Geometry check sheet. Reference: drawing and pictorial views, mm from the part's lowest x, y, z. A direction names the side the tool comes from. Coordinates: 2 decimals unless noted, no trailing zeros. Order: outer loops, then holes, each group sorted by start corner. A loop starts at its lowest first (then second) coordinate and runs counter-clockwise, first axis right, second up. Notation, with made-up numbers: (18.5, 58.25) -> (56.5, 58.25) arc R27 ccw to (56.5, 83.25) -> close; hole circle Ø4 at (75.25, 79). An arc over 180 degrees is marked (long way). Use CSV: the item, a comma, the result in double quotes. Start each with the question number.
1) Tool access check on the marked faces 1 and 2. Record the directions out of +Z, -Z, +X, -X, +Y, -Y that give a thin tool (end or side, any length) a straight path to the whole face; none if there is none.
2) Scan lines: line 1 along X through (y, z) = (6.25, 72) (3 decimals); line 2 along Z through (x, y) = (22.5, 13.5) (3 decimals). Record each from-to range of solid material in increasing order.
3) Go/stop test with flat-tipped pins: pin 1 (12 mm diameter, centred on x = 52.5, y = 12, fed in from -Z) (3 decimals); pin 2 (5 mm diameter, centred on y = 4, z = 66, fed in from +X) (3 decimals). Record where each tip stops, or that it passes through.
4) Sectioned sample at A-A on y = 12.7. Record the boundary of the cut face in (x, z) (1 decimal).
5) Sectioned sample at B-B on x = 8. Record the boundary of the cut face in (y, z) (3 decimals).
6) Sectioned sample at C-C on z = 47. Record the boundary of the cut face in (x, y) (3 decimals).
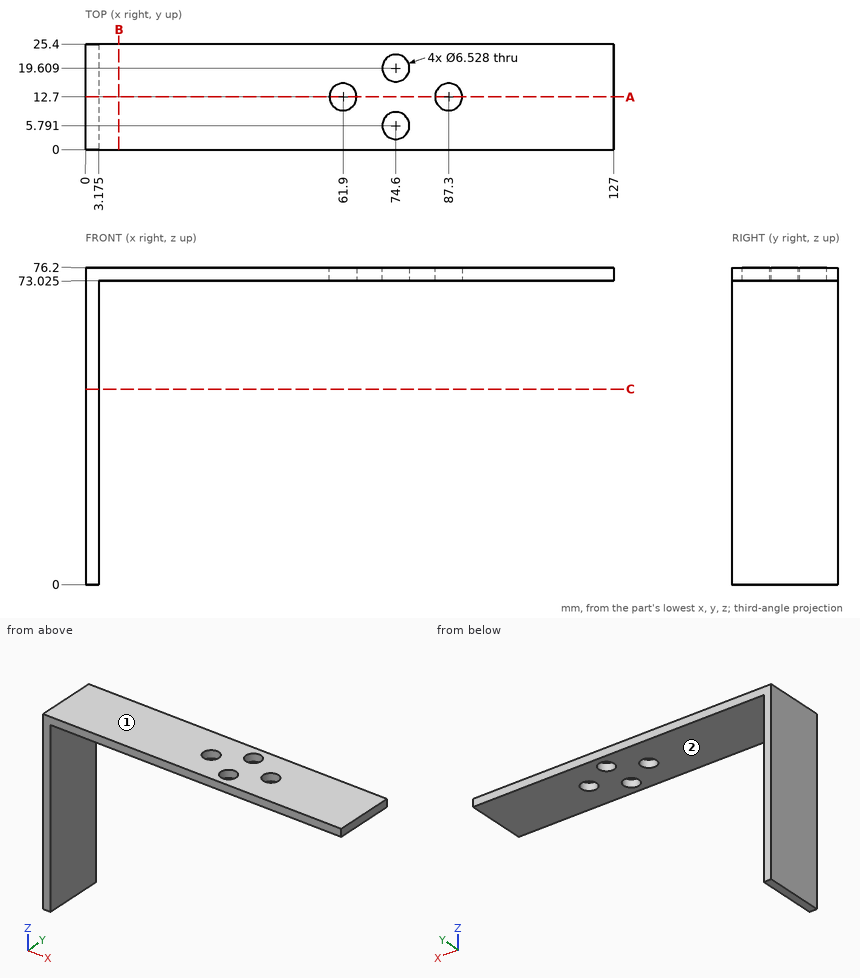
Answers follow:
1,face 1,"+Z, +X, -X, +Y, -Y"
1,face 2,"-Z, +X, +Y, -Y"
2,line 1,"x = 0 to 3.175"
2,line 2,"z = 73.025 to 76.2"
3,pin 1,"stops at z = 73.025"
3,pin 2,"stops at x = 3.175"
4,outline,"(0, 0) -> (3.2, 0) -> (3.2, 73) -> (58.6, 73) -> (58.6, 76.2) -> (0, 76.2) -> close; (65.2, 73) -> (84, 73) -> (84, 76.2) -> (65.2, 76.2) -> close; (90.6, 73) -> (127, 73) -> (127, 76.2) -> (90.6, 76.2) -> close"
5,outline,"(0, 73.025) -> (25.4, 73.025) -> (25.4, 76.2) -> (0, 76.2) -> close"
6,outline,"(0, 0) -> (3.175, 0) -> (3.175, 25.4) -> (0, 25.4) -> close"
